Verification items for the finished model (mm, model axes). Face numbers are marked on the shaded views. Coordinates: 2 decimals unless noted, no trailing zeros. Write each loop counter-clockwise with the first axis right and the second up, starting at its lowest first coordinate (ties: lowest second). Pieces come first, ordered by that corner, then holes. Notation, with made-up numbers: (42.5, 84) -> (69.5, 84) arc R18 cw to (69.5, 109) -> close; hole circle Ø11 at (78, -16). An arc over 180 degrees is marked (long way). Answer in a Markdown table with one row per item.
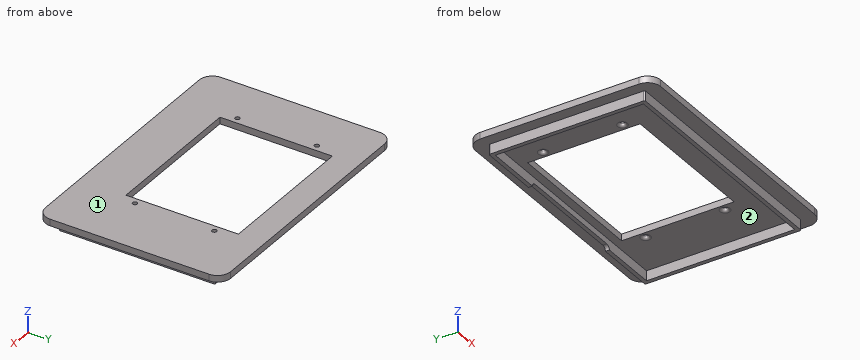
```python
from build123d import *

# Parameters (mm, degrees)
F0_W     = 200
F0_H     = 140
F0_W_2   = 183
F0_H_2   = 118
F0_W_3   = 177
F0_H_3   = 112
F0_R     = 1.75
F0_W_4   = 110
F0_H_4   = 85
F1_DEPTH = 5
F2_DEPTH = 7.5
F3_R     = 10
F4_R     = 1
F5_R     = 2
F6_W     = 45
F6_H     = 3
F7_DEPTH = 25
F8_R     = 2.99999


# Not quite as in the source:
# - a fillet or chamfer is up to 0.001 mm smaller than in the source, because OpenCascade refuses the exact size


with BuildPart() as f1:
    # F0 (on Top) → F1 (new body)
    with BuildSketch(Plane.XY):
        Rectangle(F0_W, F0_H)
        Rectangle(F0_W_2, F0_H_2, mode=Mode.SUBTRACT)
        Rectangle(F0_W_2, F0_H_2)
        Rectangle(F0_W_3, F0_H_3, mode=Mode.SUBTRACT)
        Rectangle(F0_W_3, F0_H_3)
        with Locations((-65, -25)):
            Circle(F0_R, mode=Mode.SUBTRACT)
        with Locations((55, -25)):
            Circle(F0_R, mode=Mode.SUBTRACT)
        with Locations((-5, 7.5)):
            Rectangle(F0_W_4, F0_H_4, mode=Mode.SUBTRACT)
        with Locations((-65, 35)):
            Circle(F0_R, mode=Mode.SUBTRACT)
        with Locations((55, 35)):
            Circle(F0_R, mode=Mode.SUBTRACT)
    extrude(amount=F1_DEPTH)

    # F0 (on Top) → F2 (join)
    with BuildSketch(Plane.XY):
        Rectangle(F0_W_2, F0_H_2)
        Rectangle(F0_W_3, F0_H_3, mode=Mode.SUBTRACT)
    extrude(amount=-F2_DEPTH)

    # F3
    f3_edges = [f1.edges().sort_by_distance(p)[0] for p in [
        (-100, 70, 2.5),
        (-100, -70, 2.5),
        (100, -70, 2.5),
        (100, 70, 2.5),
    ]]
    fillet(f3_edges, radius=F3_R)

    # F4
    f4_edges = [f1.edges().sort_by_distance(p)[0] for p in [
        (-91.5, -59, -3.75),
        (91.5, -59, -3.75),
        (-91.5, 59, -3.75),
        (91.5, 59, -3.75),
    ]]
    fillet(f4_edges, radius=F4_R)

    # F5
    f5_edges = [f1.edges().sort_by_distance(p)[0] for p in [
        (-66.75, -25, 0),
        (53.25, -25, 0),
        (-66.75, 35, 0),
        (53.25, 35, 0),
    ]]
    fillet(f5_edges, radius=F5_R)

    # F6 (on face) → F7 (cut)
    with BuildSketch(Plane(origin=(0, 59, 0), x_dir=(-1, 0, 0), z_dir=(0, 1, 0))):
        with Locations((-22.5, -6)):
            Rectangle(F6_W, F6_H)
        with Locations((22.5, -6)):
            Rectangle(F6_W, F6_H)
    extrude(amount=-F7_DEPTH, mode=Mode.SUBTRACT)

    # F8 (radius 3 in the source; OpenCascade refuses exactly that, so slightly less here)
    f8_edges = [f1.edges().sort_by_distance(p)[0] for p in [
        (-45, 57.5, -4.5),
        (45, 57.5, -4.5),
    ]]
    fillet(f8_edges, radius=F8_R)


solid = f1.part
```
1. Sectioned sample at A-A, the plane y = -1.5. Record the cut outline in (x, z), and give its area (3 significant figures).
Findings below:
| item | result |
|---|---|
| outline | (-100, 0) -> (-91.5, 0) -> (-91.5, -7.5) -> (-88.5, -7.5) -> (-88.5, 0) -> (-60, 0) -> (-60, 5) -> (-100, 5) -> close; (50, 0) -> (88.5, 0) -> (88.5, -7.5) -> (91.5, -7.5) -> (91.5, 0) -> (100, 0) -> (100, 5) -> (50, 5) -> close |
| area | 495 mm² |
2. Release check for a two-part mould opening along X. For the marked faces 1 and 2 record: released by +X, released by -X, zero draft, split by the parting line, or undercut.
Findings below:
| item | result |
|---|---|
| face 1 | zero draft |
| face 2 | undercut |
3. Go/stop test with flat-tipped pins: pin 1 (2 mm diameter, centred on x = 63.5, z = -4.5, fed in from +Y); pin 2 (3 mm diameter, centred on x = 55, y = 35, fed in from -Z); pin 3 (4 mm diameter, centred on y = 12, z = -4, fed in from -X); pin 4 (4 mm diameter, centred on x = -39.5, z = -4, fed in from -Y). Record where each tip stops, or that it passes through.
Findings below:
| item | result |
|---|---|
| pin 1 | stops at y = 59 |
| pin 2 | passes through |
| pin 3 | stops at x = -91.5 |
| pin 4 | stops at y = -59 |
4. Sectioned sample at C-C, the plane y = -53. Record the cut outline in (x, z).
Findings below:
| item | result |
|---|---|
| outline | (-100, 0) -> (-91.5, 0) -> (-91.5, -7.5) -> (-88.5, -7.5) -> (-88.5, 0) -> (88.5, 0) -> (88.5, -7.5) -> (91.5, -7.5) -> (91.5, 0) -> (100, 0) -> (100, 5) -> (-100, 5) -> close |
5. Material ranges on probe 1 along Y at (x, z) = (-65, 3.1); probe 2 along X at (y, z) = (49, -1.5); probe 3 along Y at (x, z) = (-49, -6.5), recorded low to high. Write a range as from..to.
Findings below:
| item | result |
|---|---|
| probe 1 | y = -70..-26.75, -23.25..33.25, 36.75..70 |
| probe 2 | x = -91.5..-88.5, 88.5..91.5 |
| probe 3 | y = -59..-56, 56..59 |
6. Sectioned sample at D-D, the plane x = -80.5. Record the cut outline in (y, z), and give its area (3 significant figures).
Findings below:
| item | result |
|---|---|
| outline | (-70, 0) -> (-59, 0) -> (-59, -7.5) -> (-56, -7.5) -> (-56, 0) -> (56, 0) -> (56, -7.5) -> (59, -7.5) -> (59, 0) -> (70, 0) -> (70, 5) -> (-70, 5) -> close |
| area | 745 mm² |
7. Sectioned sample at B-B, the plane x = 48. Record the cut outline in (y, z), and give its area (3 significant figures).
Findings below:
| item | result |
|---|---|
| outline | (-70, 0) -> (-59, 0) -> (-59, -7.5) -> (-56, -7.5) -> (-56, 0) -> (-35, 0) -> (-35, 5) -> (-70, 5) -> close; (50, 0) -> (56, 0) -> (56, -7.5) -> (59, -7.5) -> (59, 0) -> (70, 0) -> (70, 5) -> (50, 5) -> close |
| area | 320 mm² |
